```python
from build123d import *

# Parameters (mm, degrees)
SKETCH1_R           = 22.5
BOSS_EXTRUDE1_DEPTH = 3
SKETCH2_R           = 17.5
BOSS_EXTRUDE2_DEPTH = 6
CHAMFER1_SIZE       = 6
CHAMFER1_SIZE_2     = 0.5
CUT_EXTRUDE1_REACH  = 35.068
FILLET1_R           = 100
CUT_EXTRUDE2_REACH  = 35.068
SKETCH4_W           = 6.5
SKETCH4_H           = 6.5
CUT_EXTRUDE3_START  = -2
SKETCH6_R           = 22.5
SKETCH6_R_2         = 17.5
CUT_EXTRUDE3_DEPTH  = 2
CUT_EXTRUDE4_REACH  = 34.81
CIRPATTERN1_COUNT   = 6


with BuildPart() as part:
    # Sketch1 → Boss-Extrude1 (new body)
    with BuildSketch(Plane.XY):
        Circle(SKETCH1_R)
    extrude(amount=BOSS_EXTRUDE1_DEPTH)

    # Sketch2 → Boss-Extrude2 (add)
    with BuildSketch(Plane.XY.offset(3)):
        Circle(SKETCH2_R)
    extrude(amount=BOSS_EXTRUDE2_DEPTH)

    # Chamfer1
    # the kernel refuses this chamfer: 6, 0.5 mm, written as the material it takes off along each edge
    with BuildSketch(Plane(origin=(0, 0, 9), x_dir=(1, 0, 0), z_dir=(0, -1, 0))) as chamfer1_piece_1_section:
        Polygon((17.5, -CHAMFER1_SIZE), (17.5 - CHAMFER1_SIZE_2, 0), (17.5, 0), align=None)
    chamfer1_piece_1 = revolve(axis=Axis((0, 0, 9), (0, 0, 1)), mode=Mode.PRIVATE)
    chamfer1_piece_1 = split(chamfer1_piece_1, bisect_by=Plane(origin=(-17.303133917, 0, 3), z_dir=(0, 0, 1)), keep=Keep.TOP, mode=Mode.PRIVATE)
    add(chamfer1_piece_1, mode=Mode.SUBTRACT)

    # Sketch3 → Cut-Extrude1 (cut, up to next)
    with BuildSketch(Plane.XY.offset(9), mode=Mode.PRIVATE) as cut_extrude1_sk1:
        with BuildLine():
            ThreePointArc((0, 5.5), (9.191338757, 6.81195468), (15.5, 0))
            ThreePointArc((15.5, 0), (14.159954593, 6.304417968), (10.371524399, 11.518744795))
            ThreePointArc((10.371524399, 11.518744795), (1.087937204, 11.388583202), (-4.08729654, 3.680218335))
            ThreePointArc((-4.08729654, 3.680218335), (-2.237051537, 5.024500017), (0, 5.5))
        make_face()
    cut_extrude1_tool1 = extrude(cut_extrude1_sk1.sketch, amount=-CUT_EXTRUDE1_REACH, mode=Mode.PRIVATE) & part.part
    # Sketch3 → Cut-Extrude1 (cut, up to next)
    with BuildSketch(Plane.XY.offset(9), mode=Mode.PRIVATE) as cut_extrude1_sk2:
        with BuildLine():
            ThreePointArc((14.159954593, -6.304417968), (11.167377351, 2.484575984), (2.237051537, 5.024500017))
            ThreePointArc((2.237051537, 5.024500017), (4.08729654, 3.680218335), (5.23081084, 1.699593469))
            ThreePointArc((5.23081084, 1.699593469), (9.318833764, -6.636472858), (4.789763413, -14.741376003))
            ThreePointArc((4.789763413, -14.741376003), (10.371524399, -11.518744795), (14.159954593, -6.304417968))
        make_face()
    cut_extrude1_tool2 = extrude(cut_extrude1_sk2.sketch, amount=-CUT_EXTRUDE1_REACH, mode=Mode.PRIVATE) & part.part
    # Sketch3 → Cut-Extrude1 (cut, up to next)
    with BuildSketch(Plane.XY.offset(9), mode=Mode.PRIVATE) as cut_extrude1_sk3:
        with BuildLine():
            ThreePointArc((-5.23081084, 1.699593469), (-3.63827401, 10.84649238), (4.789763413, 14.741376003))
            ThreePointArc((4.789763413, 14.741376003), (-1.620191181, 15.415089378), (-7.75, 13.423393759))
            ThreePointArc((-7.75, 13.423393759), (-10.494995181, 4.553955519), (-4.763139721, -2.75))
            ThreePointArc((-4.763139721, -2.75), (-5.469870425, -0.574906548), (-5.23081084, 1.699593469))
        make_face()
    cut_extrude1_tool3 = extrude(cut_extrude1_sk3.sketch, amount=-CUT_EXTRUDE1_REACH, mode=Mode.PRIVATE) & part.part
    # Sketch3 → Cut-Extrude1 (cut, up to next)
    with BuildSketch(Plane.XY.offset(9), mode=Mode.PRIVATE) as cut_extrude1_sk4:
        with BuildLine():
            ThreePointArc((-1.620191181, -15.415089378), (5.813881563, -9.853030796), (5.469870425, -0.574906548))
            ThreePointArc((5.469870425, -0.574906548), (4.763139721, -2.75), (3.232818888, -4.449593469))
            ThreePointArc((3.232818888, -4.449593469), (-3.431982756, -10.913520471), (-12.539763413, -9.110671411))
            ThreePointArc((-12.539763413, -9.110671411), (-7.75, -13.423393759), (-1.620191181, -15.415089378))
        make_face()
    cut_extrude1_tool4 = extrude(cut_extrude1_sk4.sketch, amount=-CUT_EXTRUDE1_REACH, mode=Mode.PRIVATE) & part.part
    # Sketch3 → Cut-Extrude1 (cut, up to next)
    with BuildSketch(Plane.XY.offset(9), mode=Mode.PRIVATE) as cut_extrude1_sk5:
        with BuildLine():
            ThreePointArc((-3.232818888, -4.449593469), (-11.439915756, -0.10845373), (-12.539763413, 9.110671411))
            ThreePointArc((-12.539763413, 9.110671411), (-15.161287811, 3.222631208), (-15.161287811, -3.222631208))
            ThreePointArc((-15.161287811, -3.222631208), (-7.574200938, -8.574083908), (1.143514299, -5.379811804))
            ThreePointArc((1.143514299, -5.379811804), (-1.143514299, -5.379811804), (-3.232818888, -4.449593469))
        make_face()
    cut_extrude1_tool5 = extrude(cut_extrude1_sk5.sketch, amount=-CUT_EXTRUDE1_REACH, mode=Mode.PRIVATE) & part.part
    add(cut_extrude1_tool1.solids().sort_by_distance((5.79241, 8.44736, 9))[0], mode=Mode.SUBTRACT)
    add(cut_extrude1_tool2.solids().sort_by_distance((9.82387, -2.898532, 9))[0], mode=Mode.SUBTRACT)
    add(cut_extrude1_tool3.solids().sort_by_distance((-6.243964, 8.119288, 9))[0], mode=Mode.SUBTRACT)
    add(cut_extrude1_tool4.solids().sort_by_distance((0.279075, -10.238752, 9))[0], mode=Mode.SUBTRACT)
    add(cut_extrude1_tool5.solids().sort_by_distance((-9.651392, -3.429365, 9))[0], mode=Mode.SUBTRACT)

    # Fillet1
    fillet1_edges = [part.edges().sort_by_distance(p)[0] for p in [
        (3.232818888, -4.449593469, 4.5),
        (5.23081084, 1.699593469, 4.5),
        (-5.23081084, 1.699593469, 4.5),
        (-3.232818888, -4.449593469, 4.5),
        (0, 5.5, 4.5),
    ]]
    fillet(fillet1_edges, radius=FILLET1_R)

    # Sketch4 → Cut-Extrude2 (cut, up to next)
    with BuildSketch(Plane.XY.offset(9), mode=Mode.PRIVATE) as cut_extrude2_sk1:
        Rectangle(SKETCH4_W, SKETCH4_H)
    cut_extrude2_tool1 = extrude(cut_extrude2_sk1.sketch, amount=-CUT_EXTRUDE2_REACH, mode=Mode.PRIVATE) & part.part
    add(cut_extrude2_tool1.solids().sort_by_distance((0, 0, 9))[0], mode=Mode.SUBTRACT)

    # Sketch6 → Cut-Extrude3 (cut)
    with BuildSketch(Plane.XY.offset(3).offset(CUT_EXTRUDE3_START)):
        Circle(SKETCH6_R)
        Circle(SKETCH6_R_2, mode=Mode.SUBTRACT)
    extrude(amount=CUT_EXTRUDE3_DEPTH, mode=Mode.SUBTRACT)

    # Sketch7 → Cut-Extrude4 (cut, up to next)
    with BuildSketch(Plane.XY.offset(1), mode=Mode.PRIVATE) as cut_extrude4_sk1:
        with BuildLine():
            Line((3.73343582, 21.17336669), (-3.73343582, 21.17336669))
            Line((-3.73343582, 21.17336669), (-3.038843109, 17.234135678))
            ThreePointArc((-3.038843109, 17.234135678), (0, 17.5), (3.038843109, 17.234135678))
            Line((3.038843109, 17.234135678), (3.73343582, 21.17336669))
        make_face()
    cut_extrude4_tool1 = extrude(cut_extrude4_sk1.sketch, amount=-CUT_EXTRUDE4_REACH, mode=Mode.PRIVATE) & part.part
    # Sketch7 → Cut-Extrude4 (cut, up to next)
    with BuildSketch(Plane.XY.offset(1), mode=Mode.PRIVATE) as cut_extrude4_sk2:
        with BuildLine():
            ThreePointArc((3.73343582, 21.17336669), (0, 21.5), (-3.73343582, 21.17336669))
            Line((-3.73343582, 21.17336669), (3.73343582, 21.17336669))
        make_face()
    cut_extrude4_tool2 = extrude(cut_extrude4_sk2.sketch, amount=-CUT_EXTRUDE4_REACH, mode=Mode.PRIVATE) & part.part
    cut_extrude4_1 = cut_extrude4_tool1.solids().sort_by_distance((0, 19.352452, 1))[0]
    add(cut_extrude4_1, mode=Mode.SUBTRACT)
    cut_extrude4_2 = cut_extrude4_tool2.solids().sort_by_distance((0, 21.304105, 1))[0]
    add(cut_extrude4_2, mode=Mode.SUBTRACT)
    cut_extrude4 = cut_extrude4_1 + cut_extrude4_2  # Cut-Extrude4 as one shape, for the pattern or mirror that repeats it

    # CirPattern1: Cut-Extrude4 ×6 about axis
    cirpattern1_axis = Axis((0, 0, 0), (0, 0, 1))
    for i in range(1, CIRPATTERN1_COUNT):
        add(cut_extrude4.rotate(cirpattern1_axis, i * 360 / CIRPATTERN1_COUNT), mode=Mode.SUBTRACT)


solid = part.part
```
Here's how the part is built. I have some questions about the finished solid (model axes, mm). A direction names the side the tool comes from. Give positions to 0.01 mm unless a question says otherwise; leave off trailing zeros. Use CSV: the item, a comma, the result in double quotes. Start each with the question number.
Item 1: I'm going to push flat-ended pins straight in: P1, Ø1.5, axis at y = -7.5, z = 4.5, coming from the -X side; P2, Ø1.5, axis at x = 14.5, y = -12.5, coming from the +Z side; P3, Ø4, axis at x = 10.5, y = -9, coming from the +Z side; P4, Ø5, axis at x = 1.5, z = 3, coming from the +Y side. Where does each tip first touch, or does it pass through?
Item 2: If I drill on probe 1 along X at (y, z) = (-12.5, 8); probe 2 along Y at (x, z) = (12, 2.25); probe 3 along Y at (x, z) = (4, 7.5), over which ranges is the centre line in solid material (lowest first)? Write a range as [from, to].
Item 3: On a 3-axis mill with a long thin cutter (end or side, diameter ignored), from which of +Z, -Z, +X, -X, +Y, -Y can I reach the whole of each face in a straight line? I mean faces 4 (the conical face through (16.344, 5.147, 7.375)), 5 (the cylindrical face through (18.65, 10.7, 0.51)). Say none if no direction works.
Item 4: Suppose I cut it at A-A (x = 11.5). Give the number of separate pieces and of enclosed holes in the cut face, and give its area (3 significant figures).
Item 5: Thinking about a two-plate mould opening in Y: for faces 1 (the flat face through (0, -4, 9)), 2 (the cylindrical face through (-3.065, 4.567, 4.563)), 3 (the cylindrical face through (10.382, -19.961, 0.493)), which applies, pulls with the +Y half, pulls with the -Y half, needs draft (parallel to the pull), parting line crosses it, or undercut?
Answer block:
1,P1,"stops at x = -16.02"
1,P2,"stops at z = 1"
1,P3,"stops at z = 9"
1,P4,"stops at y = 22.5"
2,probe 1,"x = [-11.64, -9.17], [3.97, 7.22], [9.17, 11.64]"
2,probe 2,"y = [-12.74, -9.81], [1.59, 5.27], [9.81, 12.74]"
2,probe 3,"y = [-16.65, -12.47], [-3.89, 3.77], [5.23, 7.22], [12.42, 14.75], [14.97, 16.65]"
3,face 4,"+Z"
3,face 5,"+Z, -Z"
4,separate pieces,"3"
4,enclosed holes,"0"
4,area,"90.0 mm^2"
5,face 1,"needs draft"
5,face 2,"undercut"
5,face 3,"parting line crosses it"
